CAD build for the part. Positions are in the model's coordinates, mm. Face numbers are marked on the shaded views. A direction names the side the tool comes from. Coordinates: 2 decimals unless noted, no trailing zeros. Write each loop counter-clockwise with the first axis right and the second up, starting at its lowest first coordinate (ties: lowest second). Pieces come first, ordered by that corner, then holes. Notation, with made-up numbers: (11.25, -24.75) - (47.25, -24.75) arc R18 ccw to (47.25, -9.75) - close; hole circle Ø6 at (30, 58.5). An arc over 180 degrees is marked (long way). Answer in a Markdown table with one row per item. Add a question column.
Q1. Pin check, flat tips, straight feed: pin 1 (18.5 mm diameter, centred on x = 0, y = 28, fed in from -Z); pin 2 (1 mm diameter, centred on y = 34, z = 32, fed in from +X); pin 3 (1 mm diameter, centred on y = 1.5, z = 27, fed in from +X); pin 4 (1.5 mm diameter, centred on x = 35.5, z = 26, fed in from +Y). Stop position of each tip, or through.
Q2. Band-saw the part on C-C (z = 23). List the corners of the cut face in (x, y).
Q3. Band-saw the part on A-A (x = 0). List the corners of the cut face in (y, z).
Q4. Band-saw the part on D-D (x = 35). List the corners of the cut face in (y, z) (3 decimals), and give its area (3 significant figures).
Q5. Two-plate mould, pull along X, no slides. Class the marked faces 1, 2, 3 and 4: +X half, -X half, draft (parallel to the pull), parting line (faces both ways), or undercut.
Q6. Drill centre lines: line 1 along Z through (x, y) = (-3, 19); line 2 along Y through (x, z) = (0, 32.25); line 3 along X through (y, z) = (-9.5, 20). Where is each one in solid material? Low to high. Write a range as from..to.
Q7. 3-axis set-ups, long thin cutter, end or side, ignore diameter. For the marked faces 5, 6 and 7: which of +Z, -Z, +X, -X, +Y, -Y reach the whole face in a straight line?
Q8. Band-saw the part on B-B (y = 17.5). List the corners of the cut face in (x, z).
```python
from build123d import *

# Parameters (mm, degrees)
BOSS_EXTRUDE3_DEPTH     = 40
CUT_EXTRUDE4_DEPTH      = 12
CUT_EXTRUDE5_DEPTH      = 22.5
CUT_EXTRUDE7_DEPTH      = 45
SKETCH13_R              = 8
CUT_EXTRUDE8_DEPTH      = 45
CUT_EXTRUDE9_DEPTH      = 54
CUT_EXTRUDE9_DEPTH_BACK = 41
SKETCH14_R              = 8


with BuildPart() as part:
    # Sketch1 → Boss-Extrude3 (new body)
    with BuildSketch(Plane.XY):
        with BuildLine():
            Line((23, 0), (60, 0))
            Line((60, 0), (60, -12))
            Line((60, -12), (-8, -12))
            Line((-8, -12), (-8, -52))
            Line((-8, -52), (-20, -52))
            Line((-20, -52), (-20, 28))
            ThreePointArc((-20, 28), (0, 48), (20, 28))
            Line((20, 28), (20, 3))
            ThreePointArc((20, 3), (20.878679656, 0.878679656), (23, 0))
        make_face()
    extrude(amount=BOSS_EXTRUDE3_DEPTH)

    # Sketch10 → Cut-Extrude4 (cut)
    with BuildSketch(Plane(origin=(0, 0, 0), x_dir=(1, 0, 0), z_dir=(0, 1, 0))):
        with BuildLine():
            Line((60, -40), (60, -20))
            ThreePointArc((60, -20), (54.142135624, -34.142135624), (40, -40))
            Line((40, -40), (60, -40))
        make_face()
        with BuildLine():
            Line((60, -20), (60, 0))
            Line((60, 0), (40, 0))
            ThreePointArc((40, 0), (54.142135624, -5.857864376), (60, -20))
        make_face()
    extrude(amount=-CUT_EXTRUDE4_DEPTH, mode=Mode.SUBTRACT)

    # Sketch11 → Cut-Extrude5 (cut, symmetric)
    with BuildSketch(Plane(origin=(0, 0, 0), x_dir=(0, 0, -1), z_dir=(1, 0, 0))):
        Polygon((-20, 48), (-28, 48), (-28, 3), (-12, 3), (-12, 48), align=None)
    extrude(amount=CUT_EXTRUDE5_DEPTH, both=True, mode=Mode.SUBTRACT)

    # Sketch12 → Cut-Extrude7 (cut)
    with BuildSketch(Plane(origin=(-8, 0, 0), x_dir=(0, 0, -1), z_dir=(1, 0, 0))):
        with BuildLine():
            ThreePointArc((-20, -24), (-28, -32), (-20, -40))
            Line((-20, -40), (-20, -24))
        make_face()
        with BuildLine():
            Line((-20, -24), (-20, -40))
            ThreePointArc((-20, -40), (-14.343145751, -37.656854249), (-12, -32))
            ThreePointArc((-12, -32), (-14.343145751, -26.343145751), (-20, -24))
        make_face()
        with BuildLine():
            Line((-40, -52), (-20, -52))
            ThreePointArc((-20, -52), (-34.142135624, -46.142135624), (-40, -32))
            Line((-40, -32), (-40, -52))
        make_face()
        with BuildLine():
            ThreePointArc((0, -32), (-5.857864376, -46.142135624), (-20, -52))
            Line((-20, -52), (0, -52))
            Line((0, -52), (0, -32))
        make_face()
    extrude(amount=-CUT_EXTRUDE7_DEPTH, mode=Mode.SUBTRACT)

    # Sketch13 → Cut-Extrude8 (cut)
    with BuildSketch(Plane(origin=(0, 0, 0), x_dir=(1, 0, 0), z_dir=(0, 1, 0))):
        with Locations(Location((40, -20, 0), (0, 0, 270))):
            Circle(SKETCH13_R)
    extrude(amount=-CUT_EXTRUDE8_DEPTH, mode=Mode.SUBTRACT)

    # Sketch14 → Cut-Extrude9 (cut, two sides: drawn at the far end of the back side and taken through both)
    with BuildSketch(Plane.XY.offset(-CUT_EXTRUDE9_DEPTH_BACK)):
        with Locations(Location((0, 28, 0), (0, 0, 270))):
            Circle(SKETCH14_R)
    extrude(amount=CUT_EXTRUDE9_DEPTH + CUT_EXTRUDE9_DEPTH_BACK, mode=Mode.SUBTRACT)


solid = part.part
```
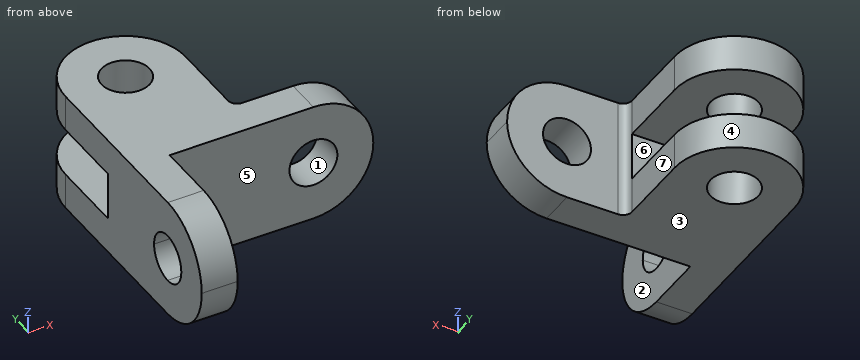
Checked values:
| question | item | result |
|---|---|---|
| 1 | pin 1 | stops at z = 0 |
| 1 | pin 2 | stops at x = 19.23 |
| 1 | pin 3 | stops at x = 20.76 |
| 1 | pin 4 | stops at y = 0 |
| 2 | outline | (-20, -51.77) - (-8, -51.77) - (-8, -39.42) - (-20, -39.42) - close; (-20, -24.58) - (-8, -24.58) - (-8, -12) - (32.58, -12) - (32.58, 0) - (23, 0) arc R3 cw to (20, 3) - (-20, 3) - close; (47.42, -12) - (59.77, -12) - (59.77, 0) - (47.42, 0) - close |
| 3 | outline | (-12, 0) - (20, 0) - (20, 12) - (3, 12) - (3, 28) - (20, 28) - (20, 40) - (-12, 40) - close; (36, 0) - (48, 0) - (48, 12) - (36, 12) - close; (36, 28) - (48, 28) - (48, 40) - (36, 40) - close |
| 4 | outline | (-12, 0) - (0, 0) - (0, 13.755) - (-12, 13.755) - close; (-12, 26.245) - (0, 26.245) - (0, 40) - (-12, 40) - close |
| 4 | area | 330 mm² |
| 5 | face 1 | undercut |
| 5 | face 2 | +X half |
| 5 | face 3 | draft |
| 5 | face 4 | parting line |
| 6 | line 1 | z = 0..12, 28..40 |
| 6 | line 2 | y = -12..20, 36..48 |
| 6 | line 3 | x = -20..32, 48..60 |
| 7 | face 5 | +Z, -Z, +X, -Y |
| 7 | face 6 | +X, -X, +Y |
| 7 | face 7 | +Z, -Z, +X, +Y |
| 8 | outline | (-20, 0) - (20, 0) - (20, 12) - (-20, 12) - close; (-20, 28) - (20, 28) - (20, 40) - (-20, 40) - close |
